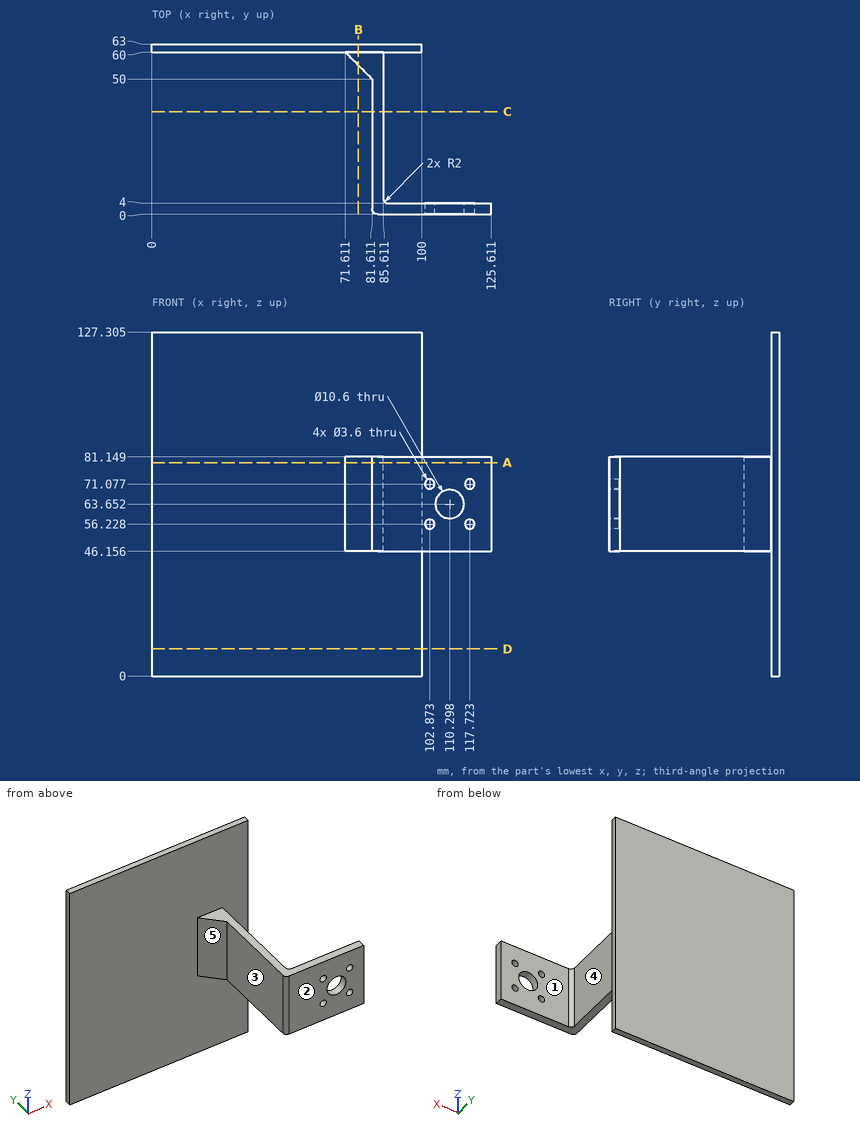
Answer from the drawing. Dimensions are ordinates in mm from the lowest x, y and z of the part. A direction names the side the tool comes from. Round coordinates to 2 decimals unless told otherwise and drop trailing zeros. Write each loop counter-clockwise with the first axis right and the second up, starting at its lowest first coordinate (ties: lowest second). Pieces come first, ordered by that corner, then holes. Notation, with made-up numbers: (6, 65.5) -> (20, 65.5) arc R25 cw to (20, 79.5) -> close; hole circle Ø8 at (-37.75, 66.5). An arc over 180 degrees is marked (long way). Answer in a Markdown table with one row per item. Add a question column.
1) Find section D-D, the plane z = 10. Determine the outline of the cut face in (x, y), and give its area (3 significant figures).
2) Find section A-A, the plane z = 79. Determine the outline of the cut face in (x, y).
3) Given P1, Ø4.5, axis at x = 102.87, z = 71.08, coming from the -Y side; P2, Ø8.5, axis at x = 110.3, z = 63.65, coming from the -Y side; P3, Ø5, axis at x = 97, z = 27, coming from the -Y side; P4, Ø10.5, axis at x = 109, z = 64.5, coming from the +Y side, each flat-ended and moving along its own axis, determine where each tip first touches the part or whether it passes through.
4) Determine the mould class of the marked faces 1, 2 and 3 for opening direction Y: pulls with the +Y half, pulls with the -Y half, needs draft (parallel to the pull), parting line crosses it, or undercut.
5) Which of the six approach directions +Z, -Z, +X, -X, +Y, -Y give full straight-line access (tool end or side, diameter ignored) to the marked faces 4 and 5?
6) Consider line 1 (Y direction, x = 62, z = 59); line 2 (X direction, y = 3.5, z = 72.5) (1 decimal); line 3 (X direction, y = 7, z = 71). Determine where each line is inside the solid, lowest interval first.
7) Find section B-B, the plane x = 76.5. Determine the outline of the cut face in (y, z) (1 decimal), and give its area (3 significant figures).
8) Find section C-C, the plane y = 38. Determine the outline of the cut face in (x, z), and give its area (3 significant figures).
Findings below:
| question | item | result |
|---|---|---|
| 1 | outline | (0, 60) -> (100, 60) -> (100, 63) -> (0, 63) -> close |
| 1 | area | 300 mm² |
| 2 | outline | (0, 60) -> (71.61, 60) -> (81.61, 50) -> (81.61, 2) arc R2 ccw to (83.61, 0) -> (125.61, 0) -> (125.61, 4) -> (87.61, 4) arc R2 cw to (85.61, 6) -> (85.61, 60) -> (100, 60) -> (100, 63) -> (0, 63) -> close |
| 3 | P1 | y = 0 |
| 3 | P2 | through |
| 3 | P3 | y = 60 |
| 3 | P4 | y = 4 |
| 4 | face 1 | undercut |
| 4 | face 2 | pulls with the -Y half |
| 4 | face 3 | needs draft |
| 5 | face 4 | +Z, -Z, +X |
| 5 | face 5 | +Z, -Z, -X, -Y |
| 6 | line 1 | 60 to 63 |
| 6 | line 2 | 81.6 to 101.8, 104 to 116.6, 118.8 to 125.6 |
| 6 | line 3 | 81.61 to 85.61 |
| 7 | outline | (55.1, 46.2) -> (60, 46.2) -> (60, 0) -> (63, 0) -> (63, 127.3) -> (60, 127.3) -> (60, 81.1) -> (55.1, 81.1) -> close |
| 7 | area | 553 mm² |
| 8 | outline | (81.61, 46.16) -> (85.61, 46.16) -> (85.61, 81.15) -> (81.61, 81.15) -> close |
| 8 | area | 140 mm² |
